Design review of the part built by this model. Coordinates are the model's own, in mm. A direction names the side the tool comes from. Round coordinates to 2 decimals unless told otherwise and drop trailing zeros. Loops run counter-clockwise (first coordinate to the right, second up) from the corner with the lowest first, then second, coordinate; pieces in that order, holes last. Notation, with made-up numbers: (17.25, -13.75) - (48.25, -13.75) arc R18 ccw to (48.25, -5.75) - close; hole circle Ø9 at (42.5, 33). An arc over 180 degrees is marked (long way). One line per question, with ' | ' between items. Start each with the question number.
from build123d import *

# Parameters (mm, degrees)
F0_R     = 7.14375
F1_DEPTH = 9.525
F3_DEPTH = 6.35
F4_R     = 4.7625
F5_DEPTH = 22.225
F6_SIZE  = 0.79375
F7_SIZE  = 0.79375
F8_SIZE  = 0.79375


with BuildPart() as f1:
    # F0 (on Top) → F1 (new body)
    with BuildSketch(Plane.XY):
        Circle(F0_R)
    extrude(amount=F1_DEPTH)

    # F2 (on face) → F3 (cut)
    with BuildSketch(Plane.XY.offset(9.525)):
        Polygon((2.291359, 3.96875), (-2.291359, 3.96875), (-4.582718, 0), (-2.291359, -3.96875), (2.291359, -3.96875), (4.582718, 0), align=None)
    extrude(amount=-F3_DEPTH, mode=Mode.SUBTRACT)

    # F4 (on face) → F5 (join)
    with BuildSketch(Plane(origin=(0, 0, 0), x_dir=(1, 0, 0), z_dir=(0, 0, -1))):
        Circle(F4_R)
    extrude(amount=F5_DEPTH)

    # F6
    f6_edges = [f1.edges().sort_by_distance(p)[0] for p in [
        (-7.14375, 0, 9.525),
    ]]
    chamfer(f6_edges, length=F6_SIZE)

    # F7
    f7_edges = [f1.edges().sort_by_distance(p)[0] for p in [
        (-7.14375, 0, 0),
    ]]
    chamfer(f7_edges, length=F7_SIZE)

    # F8
    f8_edges = [f1.edges().sort_by_distance(p)[0] for p in [
        (-4.7625, 0, -22.225),
    ]]
    chamfer(f8_edges, length=F8_SIZE)


solid = f1.part
1. Clearance check with flat-ended pins moving along their axes: P1, Ø8, axis at x = -1, z = -18.5, coming from the -Y side; P2, Ø4, axis at y = -4.5, z = -16.5, coming from the +X side; P3, Ø3, axis at y = -4.5, z = -7, coming from the +X side. State where each tip first meets the part, or that it passes through.
2. Take a section at B-B, the plane z = -9.5. Give the boundary of the cut face in (x, y) (1 decimal).
3. The part is to be moulded in two halves that separate along X. For faces 1 (the face through (3.45, 1.96, 6.39)), 2 (the face through (-0.09, -4.14, 9.525)), 3 (the face through (-3.78, 2.9, -10.57)), say which applies: pulls with the +X half, pulls with the -X half, needs draft (parallel to the pull), parting line crosses it, or undercut.
4. To check wall thickness, follow line 1 along X through (y, z) = (0, -9.5); line 2 along Z through (x, y) = (0.75, -2.5) (3 decimals); line 3 along X through (y, z) = (-3.25, 5). State the ranges of each line that lie inside material, in increasing order.
5. Machinability: for faces 4 (the face through (0, 0, -22.225)), 5 (the face through (0, 3.969, 6)), 6 (the face through (1, 5, 0)), which of the approach directions +Z, -Z, +X, -X, +Y, -Y give a long, thin tool a straight path to every point of the face, cutting with its end or side? Answer none if there is none.
Answer list:
1) P1: stops at y = -4.76 | P2: stops at x = 4.05 | P3: stops at x = 3.7
2) outline: circle Ø9.5 at (0, 0)
3) face 1: undercut | face 2: needs draft | face 3: parting line crosses it
4) line 1: x = -4.76 to 4.76 | line 2: z = -22.225 to 3.175 | line 3: x = -6.36 to -2.71, 2.71 to 6.36
5) face 4: -Z, +X, -X, +Y, -Y | face 5: +Z | face 6: -Z
